Verification items for the finished model (mm, model axes). A direction names the side the tool comes from. Give positions to 0.01 mm unless a question says otherwise; leave off trailing zeros. Write each loop counter-clockwise with the first axis right and the second up, starting at its lowest first coordinate (ties: lowest second). Pieces come first, ordered by that corner, then holes. Notation, with made-up numbers: (51, -29.5) -> (88, -29.5) arc R33 cw to (88, 2.5) -> close; hole circle Ø9 at (20.25, -0.75). An arc over 180 degrees is marked (long way). Answer as CSV lines item,"result". Start each with the question number.
1) Sectioned sample at A-A on x = 0. Record the cut outline in (y, z), and give its area (3 significant figures).
2) Mould release check, pull along X, two halves, no side actions. Record for faces 1 (the flat face through (0, 0, 0)), 2 (the flat face through (3, -15, 27)), 3 (the cylindrical face through (-2.86, -0.9, 46.41)): released by +X, released by -X, zero draft, split by the parting line, or undercut.
3) Gauge pin test, flat ends, axial feed: pin 1 Ø10 at (y, z) = (-3.5, 46.5) entering from +X; pin 2 Ø1.2 at (x, y) = (9.5, -10.5) entering from +Z; pin 3 Ø6 at (x, z) = (13.5, 22.5) entering from -Y. Record the tip position at first contact, or that the pin passes through.
4) Material ranges on L1, parallel to Z at x = -14, y = -4.5; L2, parallel to Z at x = 8, y = -3; L3, parallel to Y at x = -1.5, z = 4, recorded low to high.
5) Sectioned sample at C-C on z = 17.5. Record the cut outline in (x, y).
6) Sectioned sample at D-D on x = -6.5. Record the cut outline in (y, z).
7) Tool access check on faces 4 (the flat face through (0, 0, 53)), 5 (the cylindrical face through (-15.552, 4.572, 31.056)). Record the directions out of +Z, -Z, +X, -X, +Y, -Y that give a thin tool (end or side, any length) a straight path to the whole face; none if there is none.
```python
from build123d import *

# Parameters (mm, degrees)
ESQUISSE1_R             = 19
BOSS_EXTRU_1_DEPTH      = 35
ESQUISSE2_R             = 10
BOSS_EXTRU_2_DEPTH      = 5
ESQUISSE3_R             = 3
BOSS_EXTRU_3_DEPTH      = 13
ESQUISSE4_R             = 1.25
ENL_V_MAT_EXTRU_1_DEPTH = 8


with BuildPart() as part:
    # Esquisse1 → Boss.-Extru.1 (new body)
    with BuildSketch(Plane.XY):
        Circle(ESQUISSE1_R)
    extrude(amount=BOSS_EXTRU_1_DEPTH)

    # Esquisse2 → Boss.-Extru.2 (add)
    with BuildSketch(Plane.XY.offset(35)):
        Circle(ESQUISSE2_R)
    extrude(amount=BOSS_EXTRU_2_DEPTH)

    # Esquisse3 → Boss.-Extru.3 (add)
    with BuildSketch(Plane.XY.offset(40)):
        with Locations(Location((0, 0, 0), (0, 0, 180))):
            Circle(ESQUISSE3_R)
    extrude(amount=BOSS_EXTRU_3_DEPTH)

    # Esquisse4 → Enlèv. mat.-Extru.1 (cut)
    with BuildSketch(Plane.XY.offset(35)):
        with Locations((3.239548848, -14.646000248)):
            Circle(ESQUISSE4_R)
        with Locations((9.453296275, -10.326431598)):
            Circle(ESQUISSE4_R)
        with Locations((-13.669600231, -3.023578925)):
            Circle(ESQUISSE4_R)
        with Locations((-14.303582703, 4.517468525)):
            Circle(ESQUISSE4_R)
        with Locations((4.216303956, 13.350010522)):
            Circle(ESQUISSE4_R)
        with Locations((11.064033854, 10.128531723)):
            Circle(ESQUISSE4_R)
    extrude(amount=-ENL_V_MAT_EXTRU_1_DEPTH, mode=Mode.SUBTRACT)


solid = part.part
```
Ans:
1,outline,"(-19, 0) -> (19, 0) -> (19, 35) -> (10, 35) -> (10, 40) -> (3, 40) -> (3, 53) -> (-3, 53) -> (-3, 40) -> (-10, 40) -> (-10, 35) -> (-19, 35) -> close"
1,area,"1,510 mm²"
2,face 1,"zero draft"
2,face 2,"undercut"
2,face 3,"split by the parting line"
3,pin 1,"stops at x = 3"
3,pin 2,"stops at z = 27"
3,pin 3,"stops at y = -15.84"
4,L1,"z = 0 to 35"
4,L2,"z = 0 to 40"
4,L3,"y = -18.94 to 18.94"
5,outline,"circle Ø38 at (0, 0)"
6,outline,"(-17.85, 0) -> (17.85, 0) -> (17.85, 35) -> (7.6, 35) -> (7.6, 40) -> (-7.6, 40) -> (-7.6, 35) -> (-17.85, 35) -> close"
7,face 4,"+Z, +X, -X, +Y, -Y"
7,face 5,"+Z"
